```python
from build123d import *

# Parameters (mm, degrees)
BOARD_DEPTH            = 0.8
SKETCH2_R              = 0.5
NON_PLATED_HOLES_DEPTH = 52.351046727
SKETCH3_R              = 0.2
PLATED_HOLES_DEPTH     = 52.351046727


with BuildPart() as part:
    # Sketch1 → BOARD (new body)
    with BuildSketch(Plane.XY):
        with BuildLine():
            Line((7.65, 0), (2, 0))
            ThreePointArc((2, 0), (0.585786438, 0.585786438), (0, 2))
            Line((0, 2), (0, 17))
            ThreePointArc((0, 17), (0.585786438, 18.414213562), (2, 19))
            Line((2, 19), (7.65, 19))
            ThreePointArc((7.65, 19), (7.862132034, 18.912132034), (7.95, 18.7))
            Line((7.95, 18.7), (7.95, 18.15))
            ThreePointArc((7.95, 18.15), (8.125735931, 17.725735931), (8.55, 17.55))
            ThreePointArc((8.55, 17.55), (8.974264069, 17.725735931), (9.15, 18.15))
            Line((9.15, 18.15), (9.15, 18.7))
            ThreePointArc((9.15, 18.7), (9.237867966, 18.912132034), (9.45, 19))
            Line((9.45, 19), (17.85, 19))
            ThreePointArc((17.85, 19), (18.062132034, 18.912132034), (18.15, 18.7))
            Line((18.15, 18.7), (18.15, 18.15))
            ThreePointArc((18.15, 18.15), (18.325735931, 17.725735931), (18.75, 17.55))
            ThreePointArc((18.75, 17.55), (19.174264069, 17.725735931), (19.35, 18.15))
            Line((19.35, 18.15), (19.35, 18.7))
            ThreePointArc((19.35, 18.7), (19.437867966, 18.912132034), (19.65, 19))
            Line((19.65, 19), (28.05, 19))
            ThreePointArc((28.05, 19), (28.262132034, 18.912132034), (28.35, 18.7))
            Line((28.35, 18.7), (28.35, 18.15))
            ThreePointArc((28.35, 18.15), (28.525735931, 17.725735931), (28.95, 17.55))
            ThreePointArc((28.95, 17.55), (29.374264069, 17.725735931), (29.55, 18.15))
            Line((29.55, 18.15), (29.55, 18.7))
            ThreePointArc((29.55, 18.7), (29.637867966, 18.912132034), (29.85, 19))
            Line((29.85, 19), (38.25, 19))
            ThreePointArc((38.25, 19), (38.462132034, 18.912132034), (38.55, 18.7))
            Line((38.55, 18.7), (38.55, 18.15))
            ThreePointArc((38.55, 18.15), (38.725735931, 17.725735931), (39.15, 17.55))
            ThreePointArc((39.15, 17.55), (39.574264069, 17.725735931), (39.75, 18.15))
            Line((39.75, 18.15), (39.75, 18.7))
            ThreePointArc((39.75, 18.7), (39.837867966, 18.912132034), (40.05, 19))
            Line((40.05, 19), (45.7, 19))
            ThreePointArc((45.7, 19), (47.114213562, 18.414213562), (47.7, 17))
            Line((47.7, 17), (47.7, 2))
            ThreePointArc((47.7, 2), (47.114213562, 0.585786438), (45.7, 0))
            Line((45.7, 0), (40.05, 0))
            ThreePointArc((40.05, 0), (39.837867966, 0.087867966), (39.75, 0.3))
            Line((39.75, 0.3), (39.75, 0.85))
            ThreePointArc((39.75, 0.85), (39.574264069, 1.274264069), (39.15, 1.45))
            ThreePointArc((39.15, 1.45), (38.725735931, 1.274264069), (38.55, 0.85))
            Line((38.55, 0.85), (38.55, 0.3))
            ThreePointArc((38.55, 0.3), (38.462132034, 0.087867966), (38.25, 0))
            Line((38.25, 0), (29.85, 0))
            ThreePointArc((29.85, 0), (29.637867966, 0.087867966), (29.55, 0.3))
            Line((29.55, 0.3), (29.55, 0.85))
            ThreePointArc((29.55, 0.85), (29.374264069, 1.274264069), (28.95, 1.45))
            ThreePointArc((28.95, 1.45), (28.525735931, 1.274264069), (28.35, 0.85))
            Line((28.35, 0.85), (28.35, 0.3))
            ThreePointArc((28.35, 0.3), (28.262132034, 0.087867966), (28.05, 0))
            Line((28.05, 0), (19.65, 0))
            ThreePointArc((19.65, 0), (19.437867966, 0.087867966), (19.35, 0.3))
            Line((19.35, 0.3), (19.35, 0.85))
            ThreePointArc((19.35, 0.85), (19.174264069, 1.274264069), (18.75, 1.45))
            ThreePointArc((18.75, 1.45), (18.325735931, 1.274264069), (18.15, 0.85))
            Line((18.15, 0.85), (18.15, 0.3))
            ThreePointArc((18.15, 0.3), (18.062132034, 0.087867966), (17.85, 0))
            Line((17.85, 0), (9.45, 0))
            ThreePointArc((9.45, 0), (9.237867966, 0.087867966), (9.15, 0.3))
            Line((9.15, 0.3), (9.15, 0.85))
            ThreePointArc((9.15, 0.85), (8.974264069, 1.274264069), (8.55, 1.45))
            ThreePointArc((8.55, 1.45), (8.125735931, 1.274264069), (7.95, 0.85))
            Line((7.95, 0.85), (7.95, 0.3))
            ThreePointArc((7.95, 0.3), (7.862132034, 0.087867966), (7.65, 0))
        make_face()
    extrude(amount=BOARD_DEPTH)

    # Sketch2 → NON-PLATED HOLES (cut, through all)
    with BuildSketch(Plane.XY):
        with Locations((6.55, 17.35)):
            Circle(SKETCH2_R)
        with Locations((6.55, 1.65)):
            Circle(SKETCH2_R)
        with Locations((41.15, 17.35)):
            Circle(SKETCH2_R)
        with Locations((41.15, 1.65)):
            Circle(SKETCH2_R)
    extrude(amount=NON_PLATED_HOLES_DEPTH, mode=Mode.SUBTRACT)

    # Sketch3 → PLATED HOLES (cut, through all)
    with BuildSketch(Plane.XY):
        with Locations((37.5, 10.25)):
            Circle(SKETCH3_R)
        with Locations((26.75, 10.5)):
            Circle(SKETCH3_R)
        with Locations((14, 10)):
            Circle(SKETCH3_R)
        with Locations((30.25, 6.25)):
            Circle(SKETCH3_R)
        with Locations((31.25, 6)):
            Circle(SKETCH3_R)
        with Locations((32.5, 5.75)):
            Circle(SKETCH3_R)
        with Locations((34, 5.75)):
            Circle(SKETCH3_R)
        with Locations((33.5, 8.5)):
            Circle(SKETCH3_R)
        with Locations((35.75, 7.25)):
            Circle(SKETCH3_R)
        with Locations((21.75, 7.5)):
            Circle(SKETCH3_R)
        with Locations((22.5, 8.75)):
            Circle(SKETCH3_R)
        with Locations((29.5, 7.5)):
            Circle(SKETCH3_R)
        with Locations((28.5, 7.5)):
            Circle(SKETCH3_R)
        with Locations((27.5, 7.5)):
            Circle(SKETCH3_R)
        with Locations((26.5, 7.5)):
            Circle(SKETCH3_R)
        with Locations((29.5, 12)):
            Circle(SKETCH3_R)
        with Locations((40.75, 12.75)):
            Circle(SKETCH3_R)
        with Locations((41.75, 13.25)):
            Circle(SKETCH3_R)
        with Locations((43, 13.75)):
            Circle(SKETCH3_R)
        with Locations((44.25, 13.75)):
            Circle(SKETCH3_R)
        with Locations((45.5, 13.75)):
            Circle(SKETCH3_R)
    extrude(amount=PLATED_HOLES_DEPTH, mode=Mode.SUBTRACT)


solid = part.part
```
Input: part model. Units: mm. Frame: model coordinates. Coordinates: 2 decimals unless noted, no trailing zeros. Loops run counter-clockwise (first coordinate to the right, second up) from the corner with the lowest first, then second, coordinate; pieces in that order, holes last. Notation, with made-up numbers: M -27.75,85 L 20.25,85 A22 cw 20.25,108 Z; hole C -18.75,-11.5 d5. An arc over 180 degrees is marked long. One line per item, written item: value.
(1) Line query: line 1 along X through (y, z) = (12.75, 0.3); line 2 along X through (y, z) = (5.75, 0.5); line 3 along Y through (x, z) = (14, 0.3). Output: solid intervals per line, ascending. Write a range as from..to.
Filled in:
line 1: 0..40.55, 40.95..47.7
line 2: 0..32.3, 32.7..33.8, 34.2..47.7
line 3: 0..9.8, 10.2..19
(2) Section B-B (z = 0.55). Give the number of separate pieces and of enclosed holes in the cut face, and give its area (3 significant figures).
Filled in:
separate pieces: 1
enclosed holes: 25
area: 884 mm^2
(3) Section A-A (x = 6.55). Output: boundary loops of the cut face in (y, z), and give its area (3 significant figures).
Filled in:
outline: M 0,0 L 1.15,0 L 1.15,0.8 L 0,0.8 Z; M 2.15,0 L 16.85,0 L 16.85,0.8 L 2.15,0.8 Z; M 17.85,0 L 19,0 L 19,0.8 L 17.85,0.8 Z
area: 13.6 mm^2
(4) Pull-direction query (Y, two-part tool) for faces 1 (the cylindrical face through (47.1, 18.43, 0.39)), 2 (the cylindrical face through (7.012, 1.458, 0.394)), 3 (the flat face through (24, 10, 0.8)); classes: +Y half, -Y half, draft (parallel to the pull), parting line (faces both ways), or undercut.
Filled in:
face 1: +Y half
face 2: undercut
face 3: draft
